Can you work these out from the model? Positions are in its coordinate system, mm. A direction names the side the tool comes from. Give positions to 0.01 mm unless a question says otherwise; leave off trailing zeros. Loops run counter-clockwise (first coordinate to the right, second up) from the corner with the lowest first, then second, coordinate; pieces in that order, holes last.
from build123d import *

# Parameters (mm, degrees)
BOSS_EXTRUDE1_DEPTH    = 222.57
F_20_0MM_DOWEL_HOLE1_D = 20


with BuildPart() as part:
    # Sketch1 → Boss-Extrude1 (new body)
    with BuildSketch(Plane.XY):
        with BuildLine():
            Line((0, 0), (-110, 0))
            Line((-110, 0), (-110, -55))
            Line((-110, -55), (-85, -55))
            ThreePointArc((-85, -55), (-63.786796564, -63.786796564), (-55, -85))
            Line((-55, -85), (-55, -270))
            Line((-55, -270), (0, -270))
            Line((0, -270), (0, 0))
        make_face()
    extrude(amount=BOSS_EXTRUDE1_DEPTH)

    # Ø20.0mm Dowel Hole1 (through all)
    with Locations(Plane.XY.offset(222.57)):
        with Locations((-82.5, -27.5), (-27.5, -27.5)):
            Hole(F_20_0MM_DOWEL_HOLE1_D / 2)


solid = part.part
(1) Which directions (+Z, -Z, +X, -X, +Y, -Y) give clear straight access to the entire face, cutting with the end or side of a thin tool? Please do faces 5 (the flat face through (-55, -176, 110)), 6 (the flat face through (-44, -103, 222.57)).
Returned:
face 5: +Z, -Z, -X, -Y
face 6: +Z, +X, -X, +Y, -Y
(2) Please list where these lines run through material, in increasing order: probe 1 along Y at (x, z) = (-27, 134); probe 2 along X at (y, z) = (-27, 105); probe 3 along X at (y, z) = (-24, 142.5).
Returned:
probe 1: y = -270 to -37.49, -17.51 to 0
probe 2: x = -110 to -92.49, -72.51 to -37.49, -17.51 to 0
probe 3: x = -110 to -91.87, -73.13 to -36.87, -18.13 to 0
(3) Suppose I cut it at A-A on x = -27.5. List the corners of the cut face in (y, z) for me.
Returned:
outline: (-270, 0) - (-37.5, 0) - (-37.5, 222.57) - (-270, 222.57) - close; (-17.5, 0) - (0, 0) - (0, 222.57) - (-17.5, 222.57) - close
(4) Suppose I cut it at C-C on y = -34. List the corners of the cut face in (x, z) for me, plus the area to 3 significant figures.
Returned:
outline: (-110, 0) - (-90.1, 0) - (-90.1, 222.57) - (-110, 222.57) - close; (-74.9, 0) - (-35.1, 0) - (-35.1, 222.57) - (-74.9, 222.57) - close; (-19.9, 0) - (0, 0) - (0, 222.57) - (-19.9, 222.57) - close
area: 17,700 mm2
(5) Suppose I cut it at B-B on z = 150. List the corners of the cut face in (x, y) for me.
Returned:
outline: (-110, -55) - (-85, -55) arc R30 cw to (-55, -85) - (-55, -270) - (0, -270) - (0, 0) - (-110, 0) - close; hole circle Ø20 at (-82.5, -27.5); hole circle Ø20 at (-27.5, -27.5)
(6) Thinking about a two-plate mould opening in Y: for faces 1 (the flat face through (-54, 0, 110)), 2 (the cylindrical face through (-72.51, -27.06, 109.73)), 3 (the cylindrical face through (-36.737, -31.33, 109.727)), 4 (the flat face through (-110, -27, 110)), which applies, pulls with the +Y half, pulls with the -Y half, needs draft (parallel to the pull), parting line crosses it, or undercut?
Returned:
face 1: pulls with the +Y half
face 2: undercut
face 3: undercut
face 4: needs draft
(7) Will these pins go through, and if not, where does the flat tip stop? P1, Ø2, axis at y = -237.5, z = 160, coming from the -X side; P2, Ø8, axis at y = -69.5, z = 95.5, coming from the -X side; P3, Ø7.5, axis at x = -103.5, z = 89.5, coming from the -Y side.
Returned:
P1: stops at x = -55
P2: stops at x = -62.2
P3: stops at y = -55
(8) Suppose I cut it at D-D on y = -221.5. List the corners of the cut face in (x, z) for me.
Returned:
outline: (-55, 0) - (0, 0) - (0, 222.57) - (-55, 222.57) - close
